```python
from build123d import *

# Parameters (mm, degrees)
F0_W     = 762
F0_H     = 101.6
F0_R     = 12.7
F1_DEPTH = 6.35
F2_W     = 9.525
F2_H     = 50.8
F3_DEPTH = 6.351
F4_SIZE  = 12.7
F5_R     = 1.6002


with BuildPart() as f1:
    # F0 (on Front) → F1 (new body)
    with BuildSketch(Plane.XZ):
        with Locations((-5.1130652428, -126.3789658944)):
            Rectangle(F0_W, F0_H)
        with Locations((-322.6130652428, -126.3789658944)):
            Circle(F0_R, mode=Mode.SUBTRACT)
        with Locations((-195.6130652428, -126.3789658944)):
            Circle(F0_R, mode=Mode.SUBTRACT)
        with Locations((-68.6130652428, -126.3789658944)):
            Circle(F0_R, mode=Mode.SUBTRACT)
        with Locations((58.3869347572, -126.3789658944)):
            Circle(F0_R, mode=Mode.SUBTRACT)
        with Locations((185.3869347572, -126.3789658944)):
            Circle(F0_R, mode=Mode.SUBTRACT)
        with Locations((312.3869347572, -126.3789658944)):
            Circle(F0_R, mode=Mode.SUBTRACT)
    extrude(amount=F1_DEPTH)

    # F2 (on face) → F3 (cut, through all)
    with BuildSketch(Plane.XZ.offset(6.35)):
        with Locations((-287.6753652428, -126.3789658944)):
            Rectangle(F2_W, F2_H)
        with Locations((-274.9753652428, -126.3789658944)):
            Rectangle(F2_W, F2_H)
        with Locations((-262.2753652428, -126.3789658944)):
            Rectangle(F2_W, F2_H)
        with Locations((-249.5753652428, -126.3789658944)):
            Rectangle(F2_W, F2_H)
        with Locations((-236.8753652428, -126.3789658944)):
            Rectangle(F2_W, F2_H)
        with Locations((-160.6753652428, -126.3789658944)):
            Rectangle(F2_W, F2_H)
        with Locations((-147.9753652428, -126.3789658944)):
            Rectangle(F2_W, F2_H)
        with Locations((-135.2753652428, -126.3789658944)):
            Rectangle(F2_W, F2_H)
        with Locations((-122.5753652428, -126.3789658944)):
            Rectangle(F2_W, F2_H)
        with Locations((-109.8753652428, -126.3789658944)):
            Rectangle(F2_W, F2_H)
        with Locations((-33.6753652428, -126.3789658944)):
            Rectangle(F2_W, F2_H)
        with Locations((-20.9753652428, -126.3789658944)):
            Rectangle(F2_W, F2_H)
        with Locations((-8.2753652428, -126.3789658944)):
            Rectangle(F2_W, F2_H)
        with Locations((4.4246347572, -126.3789658944)):
            Rectangle(F2_W, F2_H)
        with Locations((17.1246347572, -126.3789658944)):
            Rectangle(F2_W, F2_H)
        with Locations((93.3246347572, -126.3789658944)):
            Rectangle(F2_W, F2_H)
        with Locations((106.0246347572, -126.3789658944)):
            Rectangle(F2_W, F2_H)
        with Locations((118.7246347572, -126.3789658944)):
            Rectangle(F2_W, F2_H)
        with Locations((131.4246347572, -126.3789658944)):
            Rectangle(F2_W, F2_H)
        with Locations((144.1246347572, -126.3789658944)):
            Rectangle(F2_W, F2_H)
        with Locations((220.3246347572, -126.3789658944)):
            Rectangle(F2_W, F2_H)
        with Locations((233.0246347572, -126.3789658944)):
            Rectangle(F2_W, F2_H)
        with Locations((245.7246347572, -126.3789658944)):
            Rectangle(F2_W, F2_H)
        with Locations((258.4246347572, -126.3789658944)):
            Rectangle(F2_W, F2_H)
        with Locations((271.1246347572, -126.3789658944)):
            Rectangle(F2_W, F2_H)
    extrude(amount=-F3_DEPTH, mode=Mode.SUBTRACT)

    # F4
    f4_edges = [f1.edges().sort_by_distance(p)[0] for p in [
        (-386.113065, -3.175, -75.578966),
        (-386.113065, -3.175, -177.178966),
        (375.886935, -3.175, -75.578966),
        (375.886935, -3.175, -177.178966),
    ]]
    chamfer(f4_edges, length=F4_SIZE)

    # F5
    f5_edges = [f1.edges().sort_by_distance(p)[0] for p in [
        (-5.113065, -6.35, -177.178966),
        (-5.113065, 0, -177.178966),
        (369.536935, -6.35, -170.828966),
        (375.886935, -6.35, -126.378966),
        (369.536935, 0, -170.828966),
        (375.886935, 0, -126.378966),
        (369.536935, -6.35, -81.928966),
        (369.536935, 0, -81.928966),
        (-5.113065, -6.35, -75.578966),
        (-5.113065, 0, -75.578966),
        (-386.113065, -6.35, -126.378966),
        (-386.113065, 0, -126.378966),
        (-379.763065, -6.35, -170.828966),
        (-379.763065, 0, -170.828966),
        (-379.763065, -6.35, -81.928966),
        (-379.763065, 0, -81.928966),
    ]]
    fillet(f5_edges, radius=F5_R)


solid = f1.part
```
Read the model definition and answer for the solid it produces. Units are mm, in the model's axes. Give positions to 0.01 mm unless a question says otherwise; leave off trailing zeros.
(1) For a pull along Z with two mould halves and no side action, classify faces 1 (the cylindrical face through (369.29, -0.46, -82.36)), 2 (the cylindrical face through (-310.88, -3.13, -131.24)), 3 (the flat face through (-10, 0, -158)), 4 (the flat face through (369.626, -3.153, -170.74)) as released by +Z, released by -Z, zero draft, split by the parting line, or undercut.
(2) Straight lines are drawn through the part: L1, parallel to Z at x = 247, y = -5.25; L2, parallel to Z at x = 12.5, y = -5; L3, parallel to Z at x = 284.5, y = -0.25. For each, find the intervals that lie inside material, in ascending order.
(3) Given pin 1 (15 mm diameter, centred on x = 185.39, z = -126.38, fed in from -Y), flat-ended and moving along its own axis, determine where the tip first touches the part or whether it passes through.
(4) Find section A-A (z = -107.5). Give the number of separate pieces and of enclosed holes in the cut face, plus the area to 3 significant figures.
Result sheet:
1. face 1: released by +Z
1. face 2: undercut
1. face 3: zero draft
1. face 4: released by -Z
2. L1: z = -177.1 to -151.78, -100.98 to -75.66
2. L2: z = -177.16 to -151.78, -100.98 to -75.6
2. L3: z = -176.44 to -76.32
3. pin 1: passes through
4. separate pieces: 26
4. enclosed holes: 0
4. area: 3,320 mm2
